The model under review builds one solid part; all positions refer to its coordinate system, in mm. Face numbers are marked on the shaded views. A direction names the side the tool comes from. Round coordinates to 2 decimals unless told otherwise and drop trailing zeros. Write each loop counter-clockwise with the first axis right and the second up, starting at its lowest first coordinate (ties: lowest second). Pieces come first, ordered by that corner, then holes. Notation, with made-up numbers: (-26.75, -37.75) -> (-18.75, -37.75) arc R13 cw to (-18.75, -13.75) -> close; hole circle Ø8 at (-28.75, 37.5). An arc over 180 degrees is marked (long way). Answer as a JSON object with one key per item and string values. Group by question number.
1) We need section A-A, the plane x = 0. Write out the cut boundary in (y, z).
2) Machinability: for the marked faces 1, 2 and 3, which of the approach directions +Z, -Z, +X, -X, +Y, -Y give a long, thin tool a straight path to every point of the face, cutting with its end or side? Answer none if there is none.
3) We need section C-C, the plane z = 0. Write out the cut boundary in (x, y).
4) Insertion check: pin 1 Ø1 at (x, y) = (-24.5, 0.5) entering from -Z; pin 2 Ø1 at (y, z) = (1.5, 16) entering from -X. Each pin has a flat end and moves straight along its axis. Give the tip position at first contact, or say it passes through.
5) To check wall thickness, follow probe 1 along X at (y, z) = (0.7, 0); probe 2 along Z at (x, y) = (-4, 1.5); probe 3 along Z at (x, y) = (-1, 0.6). State the ranges of each line that lie inside material, in increasing order. Write a range as [from, to].
6) Mouldability with a two-part tool opening along X and no side actions: class the marked faces 4, 5 and 6 as pulls with the +X half, pulls with the -X half, needs draft (parallel to the pull), parting line crosses it, or undercut.
from build123d import *

# Parameters (mm, degrees)
ESQUISSE2_R                  = 10
BOSS_EXTRU_1_DEPTH           = 2
ENL_V_MAT_EXTRU_1_REACH      = 63.767
ENL_V_MAT_EXTRU_1_END_RADIUS = 22
R_P_TITION_CIRCULAIRE1_COUNT = 4


with BuildPart() as part:
    # Esquisse2 → Boss.-Extru.1 (new body)
    with BuildSketch(Plane(origin=(0, 0, 0), x_dir=(1, 0, 0), z_dir=(0, 1, 0))):
        with BuildLine():
            Line((-1.55, 25.903667694), (-1.55, 23.5))
            ThreePointArc((-1.55, 23.5), (0, 21.95), (1.55, 23.5))
            Line((1.55, 23.5), (1.55, 25.903667694))
            ThreePointArc((1.55, 25.903667694), (4.89638147, 25.483876246), (8.160057781, 24.633634669))
            Line((8.160057781, 24.633634669), (6.917968061, 20.884006271))
            ThreePointArc((6.917968061, 20.884006271), (11, 19.052558883), (14.627095933, 16.433139219))
            Line((14.627095933, 16.433139219), (17.253324521, 19.383634669))
            ThreePointArc((17.253324521, 19.383634669), (23.348257443, 11.325253832), (25.903667694, 1.55))
            Line((25.903667694, 1.55), (23.5, 1.55))
            ThreePointArc((23.5, 1.55), (21.95, 0), (23.5, -1.55))
            Line((23.5, -1.55), (25.903667694, -1.55))
            ThreePointArc((25.903667694, -1.55), (25.483876246, -4.89638147), (24.633634669, -8.160057781))
            Line((24.633634669, -8.160057781), (20.884006271, -6.917968061))
            ThreePointArc((20.884006271, -6.917968061), (19.052558883, -11), (16.433139219, -14.627095933))
            Line((16.433139219, -14.627095933), (19.383634669, -17.253324521))
            ThreePointArc((19.383634669, -17.253324521), (11.325253832, -23.348257443), (1.55, -25.903667694))
            Line((1.55, -25.903667694), (1.55, -23.5))
            ThreePointArc((1.55, -23.5), (0, -21.95), (-1.55, -23.5))
            Line((-1.55, -23.5), (-1.55, -25.903667694))
            ThreePointArc((-1.55, -25.903667694), (-4.89638147, -25.483876246), (-8.160057781, -24.633634669))
            Line((-8.160057781, -24.633634669), (-6.917968061, -20.884006271))
            ThreePointArc((-6.917968061, -20.884006271), (-11, -19.052558883), (-14.627095933, -16.433139219))
            Line((-14.627095933, -16.433139219), (-17.253324521, -19.383634669))
            ThreePointArc((-17.253324521, -19.383634669), (-23.348257443, -11.325253832), (-25.903667694, -1.55))
            Line((-25.903667694, -1.55), (-23.5, -1.55))
            ThreePointArc((-23.5, -1.55), (-21.95, 0), (-23.5, 1.55))
            Line((-23.5, 1.55), (-25.903667694, 1.55))
            ThreePointArc((-25.903667694, 1.55), (-25.483876246, 4.89638147), (-24.633634669, 8.160057781))
            Line((-24.633634669, 8.160057781), (-20.884006271, 6.917968061))
            ThreePointArc((-20.884006271, 6.917968061), (-19.052558883, 11), (-16.433139219, 14.627095933))
            Line((-16.433139219, 14.627095933), (-19.383634669, 17.253324521))
            ThreePointArc((-19.383634669, 17.253324521), (-11.325253832, 23.348257443), (-1.55, 25.903667694))
        make_face()
        with Locations(Location((0, 0, 0), (0, 0, 270))):
            Circle(ESQUISSE2_R, mode=Mode.SUBTRACT)
    extrude(amount=BOSS_EXTRU_1_DEPTH)

    # Enlèv. mat.-Extru.1: up to this cylinder (the profile starts outside it)
    enl_v_mat_extru_1_end = Plane(origin=(0, 2.23221, 0), z_dir=(0, -1, 0)) * Cylinder(ENL_V_MAT_EXTRU_1_END_RADIUS, 172.534, mode=Mode.PRIVATE)
    # Esquisse4 → Enlèv. mat.-Extru.1 (cut, up to the surface)
    with BuildSketch(Plane(origin=(23.357789239, 0, -11.305581889), x_dir=(-0.43566789553954177, 0, -0.9001074851350516), z_dir=(0.9001074851350516, 0, -0.43566789553954177)), mode=Mode.PRIVATE) as enl_v_mat_extru_1_sk1:
        with BuildLine():
            Line((9.93063507, 1), (9.93063507, 3))
            Line((9.93063507, 3), (0, 3))
            Line((0, 3), (0, 2))
            ThreePointArc((0, 2), (0.52966098, 1.985963111), (1.057835001, 1.943891849))
            Line((1.057835001, 1.943891849), (9.93063507, 1))
        make_face()
    enl_v_mat_extru_1_tool1 = extrude(enl_v_mat_extru_1_sk1.sketch, amount=-ENL_V_MAT_EXTRU_1_REACH, mode=Mode.PRIVATE) - enl_v_mat_extru_1_end
    enl_v_mat_extru_1 = enl_v_mat_extru_1_tool1.solids().sort_by_distance((20.938912, 2.23221, -16.303079))[0]
    add(enl_v_mat_extru_1, mode=Mode.SUBTRACT)

    # Répétition circulaire1: Enlèv. mat.-Extru.1 ×4 about axis
    r_p_tition_circulaire1_axis = Axis((0, 0, 0), (0, 1, 0))
    for i in range(1, R_P_TITION_CIRCULAIRE1_COUNT):
        add(enl_v_mat_extru_1.rotate(r_p_tition_circulaire1_axis, i * 360 / R_P_TITION_CIRCULAIRE1_COUNT), mode=Mode.SUBTRACT)


solid = part.part
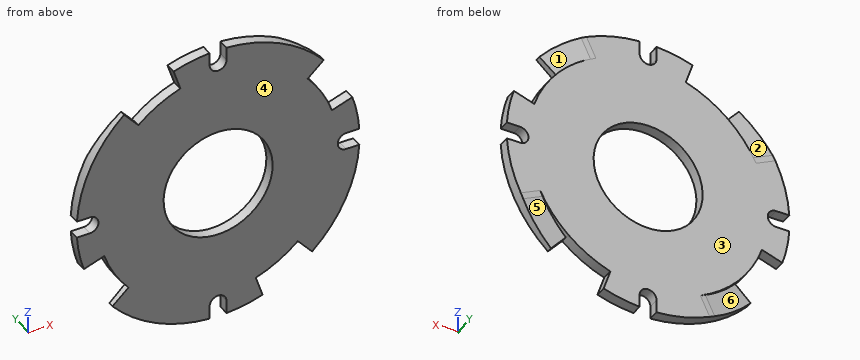
Here are the results:
{
 "1": {"outline": "(0, -21.95) -> (2, -21.95) -> (2, -10) -> (0, -10) -> close; (0, 10) -> (2, 10) -> (2, 21.95) -> (0, 21.95) -> close"},
 "2": {"face 1": "+X, +Y", "face 2": "+Z, +Y", "face 3": "+Z, -Z, +X, -X, +Y"},
 "3": {"outline": "(-21.95, 0) -> (-10, 0) -> (-10, 2) -> (-21.95, 2) -> close; (10, 0) -> (21.95, 0) -> (21.95, 2) -> (10, 2) -> close"},
 "4": {"pin 1": "stops at z = -8.16", "pin 2": "stops at x = -20.81"},
 "5": {"probe 1": "x = [-21.95, -10], [10, 21.95]", "probe 2": "z = [-25.64, -9.17], [9.17, 25.64]", "probe 3": "z = [-22.32, -9.95], [9.95, 22.32]"},
 "6": {"face 4": "needs draft", "face 5": "undercut", "face 6": "pulls with the -X half"}
}
